from build123d import *

# Parameters (mm, degrees)
ESQUISSE1_R             = 30
BASE_EXTRUSION_DEPTH    = 900
COQUE1_T                = -0.8
ENL_V_MAT_EXTRU_1_DEPTH = 100
ESQUISSE4_W             = 89
ESQUISSE4_H             = 20
BOSS_EXTRU_1_DEPTH      = 2
ESQUISSE3_R             = 6
ENL_V_MAT_EXTRU_2_DEPTH = 100


with BuildPart() as part:
    # Esquisse1 → Base-Extrusion (new body)
    with BuildSketch(Plane(origin=(0, 0, 0), x_dir=(0, 0, -1), z_dir=(1, 0, 0))):
        Circle(ESQUISSE1_R)
    extrude(amount=BASE_EXTRUSION_DEPTH)

    # Coque1
    coque1_openings = [part.faces().sort_by_distance(p)[0] for p in [
        (900, 0, 0),
        (0, 0, 0),
    ]]
    offset(amount=COQUE1_T, openings=coque1_openings, kind=Kind.INTERSECTION)

    # Esquisse2 → Enlèv. mat.-Extru.1 (cut)
    with BuildSketch(Plane(origin=(0, 0, 0), x_dir=(1, 0, 0), z_dir=(0, 1, 0))):
        with BuildLine():
            Line((-10, 23), (48, 23))
            ThreePointArc((48, 23), (63.556349186, 16.556349186), (70, 1))
            Line((70, 1), (70, -1))
            ThreePointArc((70, -1), (63.556349186, -16.556349186), (48, -23))
            Line((48, -23), (-10, -23))
            Line((-10, -23), (-10, 23))
        make_face()
    extrude(amount=ENL_V_MAT_EXTRU_1_DEPTH, mode=Mode.SUBTRACT)

    # Esquisse4 → Boss.-Extru.1 (add)
    with BuildSketch(Plane(origin=(0, 26, 0), x_dir=(-1, 0, 0), z_dir=(0, 1, 0))):
        with Locations((-115.5, 0)):
            Rectangle(ESQUISSE4_W, ESQUISSE4_H)
    extrude(amount=BOSS_EXTRU_1_DEPTH)

    # Esquisse3 → Enlèv. mat.-Extru.2 (cut)
    with BuildSketch(Plane(origin=(0, 0, 0), x_dir=(1, 0, 0), z_dir=(0, 1, 0))):
        with Locations(Location((85, 0, 0), (0, 0, 270))):
            Circle(ESQUISSE3_R)
        with Locations(Location((145, 0, 0), (0, 0, 270))):
            Circle(ESQUISSE3_R)
    extrude(amount=ENL_V_MAT_EXTRU_2_DEPTH, mode=Mode.SUBTRACT)


solid = part.part
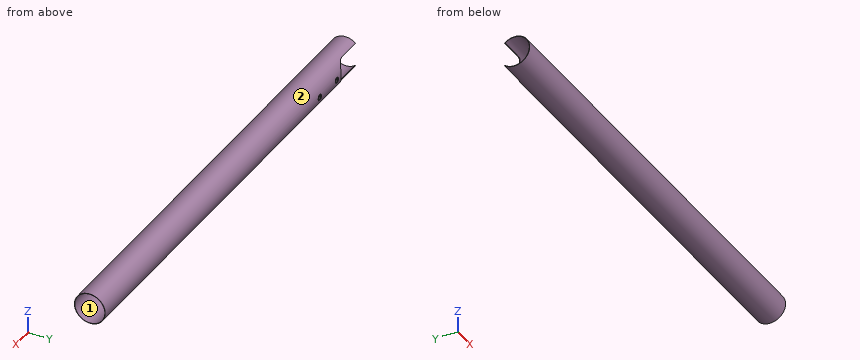
Check sheet for the modelled part. Datum: model origin and axes. Units: mm. Face numbers are marked on the shaded views. Round coordinates to 2 decimals unless told otherwise and drop trailing zeros. Loops run counter-clockwise (first coordinate to the right, second up) from the corner with the lowest first, then second, coordinate; pieces in that order, holes last.
1. Mould release check, pull along Y, two halves, no side actions. Record for the marked faces 1 and 2: released by +Y, released by -Y, zero draft, split by the parting line, or undercut.
2. Gauge pin test, flat ends, axial feed: pin 1 Ø7 at (x, z) = (145, 0) entering from +Y; pin 2 Ø1.6 at (y, z) = (26.5, -3) entering from -X; pin 3 Ø19 at (x, z) = (85, 0) entering from -Y; pin 4 Ø13.5 at (x, z) = (108, -1.5) entering from +Y. Record the tip position at first contact, or that the pin passes through.
3. Sectioned sample at A-A on y = 0. Record the boundary of the cut face in (x, z).
4. Sectioned sample at C-C on x = 61. Record the boundary of the cut face in (y, z), and give its area (3 significant figures).
5. Sectioned sample at B-B on x = 733. Record the boundary of the cut face in (y, z), and give its area (3 significant figures).
6. Scan lines: probe 1 along X at (y, z) = (29.65, 0); probe 2 along X at (y, z) = (27, 0); probe 3 along Y at (x, z) = (133, -4). Record each from-to range of solid material in increasing order.
Recorded:
1. face 1: undercut
1. face 2: split by the parting line
2. pin 1: stops at y = -28.99
2. pin 2: stops at x = 71
2. pin 3: stops at y = -30
2. pin 4: stops at y = 30
3. outline: (0, -30) - (900, -30) - (900, -29.2) - (0, -29.2) - close; (0, 29.2) - (900, 29.2) - (900, 30) - (0, 30) - close
4. outline: (22.39, -18.75) arc R29.2 cw (long way) to (22.39, 18.75) - (23.42, 18.75) arc R30 ccw (long way) to (23.42, -18.75) - close
4. area: 116 mm2
5. outline: circle Ø60 at (0, 0); hole circle Ø58.4 at (0, 0)
5. area: 149 mm2
6. probe 1: x = 70 to 79, 91 to 139, 151 to 900
6. probe 2: x = 71 to 79, 91 to 139, 151 to 160
6. probe 3: y = -29.73 to -28.92, 26 to 28, 28.92 to 29.73
